Geometry: see drawing. Coordinates: mm, zero at the bounding-box minimum. Coordinates: 2 decimals unless noted, no trailing zeros. Order: outer loops, then holes, each group sorted by start corner. A loop starts at its lowest first (then second) coordinate and runs counter-clockwise, first axis right, second up.
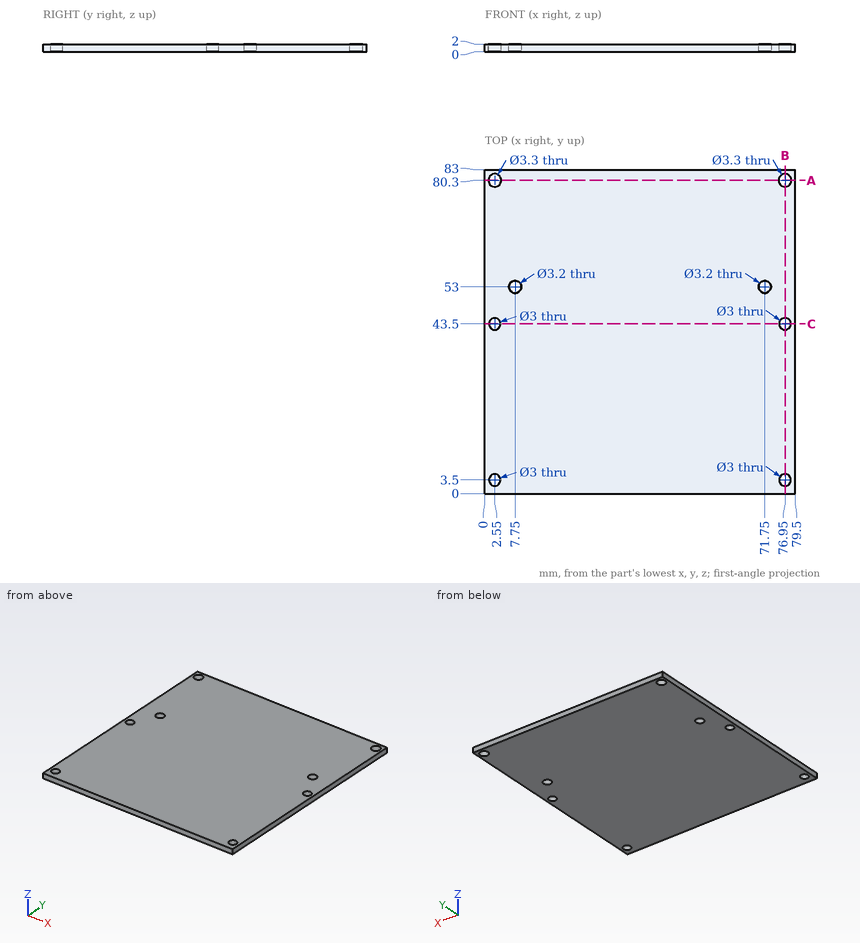
Q1. Section query A-A on y = 80.3. Output: boundary loops of the cut face in (x, z), plus the area to 3 significant figures.
Solutions:
outline: (0, 0) - (0.9, 0) - (0.9, 2) - (0, 2) - close; (4.2, 0) - (75.3, 0) - (75.3, 2) - (4.2, 2) - close; (78.6, 0) - (79.5, 0) - (79.5, 2) - (78.6, 2) - close
area: 146 mm2
Q2. Pin query (flat end, axial travel): P1, Ø3.5, axis at x = 7.75, y = 53, coming from the -Z side; P2, Ø2, axis at x = 2.55, y = 80.3, coming from the +Z side. Return the tip coordinate at first contact, or that it passes through.
Solutions:
P1: stops at z = 0
P2: passes through
Q3. Section query C-C on y = 43.5. Output: boundary loops of the cut face in (x, z), plus the area to 3 significant figures.
Solutions:
outline: (0, 0) - (1.05, 0) - (1.05, 2) - (0, 2) - close; (4.05, 0) - (75.45, 0) - (75.45, 2) - (4.05, 2) - close; (78.45, 0) - (79.5, 0) - (79.5, 2) - (78.45, 2) - close
area: 147 mm2
Q4. Section query B-B on x = 76.95. Output: boundary loops of the cut face in (y, z).
Solutions:
outline: (0, 0) - (2, 0) - (2, 2) - (0, 2) - close; (5, 0) - (42, 0) - (42, 2) - (5, 2) - close; (45, 0) - (78.65, 0) - (78.65, 2) - (45, 2) - close; (81.95, 0) - (83, 0) - (83, 2) - (81.95, 2) - close
Q5. Material intervals for line 1 along X through (y, z) = (3.5, 0.8); line 2 along Y through (x, z) = (2.55, 1.45); line 3 along X through (y, z) = (53, 1.25), sorted ascending.
Solutions:
line 1: x = 0 to 1.05, 4.05 to 75.45, 78.45 to 79.5
line 2: y = 0 to 2, 5 to 42, 45 to 78.65, 81.95 to 83
line 3: x = 0 to 6.15, 9.35 to 70.15, 73.35 to 79.5
